Design review of the part built by this model. Coordinates are the model's own, in mm. Coordinates: 2 decimals unless noted, no trailing zeros. Use a Markdown table: item, result.
from build123d import *

# Parameters (mm, degrees)
F0_R     = 47.625
F0_R_2   = 1.5875
F0_R_3   = 19.05
F0_R_4   = 14.2875
F1_DEPTH = 3.175
F2_DEPTH = 12.7
F3_SIZE  = 3.17499
F4_SIZE  = 0.79375
F5_SIZE  = 0.79375
F6_R     = 5.08
F7_SIZE  = 3.175


# Not quite as in the source:
# - a fillet or chamfer is up to 0.001 mm smaller than in the source, because OpenCascade refuses the exact size


with BuildPart() as f1:
    # F0 (on Front) → F1 (new body)
    with BuildSketch(Plane.XZ):
        Circle(F0_R)
        with Locations((0, -34.925)):
            Circle(F0_R_2, mode=Mode.SUBTRACT)
        with Locations((-34.925, 0)):
            Circle(F0_R_2, mode=Mode.SUBTRACT)
        Circle(F0_R_3, mode=Mode.SUBTRACT)
        with Locations((34.925, 0)):
            Circle(F0_R_2, mode=Mode.SUBTRACT)
        with Locations((0, 34.925)):
            Circle(F0_R_2, mode=Mode.SUBTRACT)
        Circle(F0_R_3)
        Circle(F0_R_4, mode=Mode.SUBTRACT)
    extrude(amount=F1_DEPTH)

    # F0 (on Front) → F2 (join)
    with BuildSketch(Plane.XZ):
        Circle(F0_R_3)
        Circle(F0_R_4, mode=Mode.SUBTRACT)
    extrude(amount=F2_DEPTH)

    # F3 (size 3.175 in the source; OpenCascade refuses exactly that, so slightly less here)
    f3_edges = [f1.edges().sort_by_distance(p)[0] for p in [
        (-1.5875, -3.175, 34.925),
        (-36.5125, -3.175, 0),
        (33.3375, -3.175, 0),
        (-1.5875, -3.175, -34.925),
    ]]
    chamfer(f3_edges, length=F3_SIZE)

    # F4
    f4_edges = [f1.edges().sort_by_distance(p)[0] for p in [
        (-47.625, -3.175, 0),
    ]]
    chamfer(f4_edges, length=F4_SIZE)

    # F5
    f5_edges = [f1.edges().sort_by_distance(p)[0] for p in [
        (-19.05, -12.7, 0),
        (-14.2875, -12.7, 0),
    ]]
    chamfer(f5_edges, length=F5_SIZE)

    # F6
    f6_edges = [f1.edges().sort_by_distance(p)[0] for p in [
        (-19.05, -3.175, 0),
    ]]
    fillet(f6_edges, radius=F6_R)

    # F7
    f7_edges = [f1.edges().sort_by_distance(p)[0] for p in [
        (-14.2875, 0, 0),
    ]]
    chamfer(f7_edges, length=F7_SIZE)


solid = f1.part
(1) For pin 1 (2.5 mm diameter, centred on x = -34.925, z = 0, fed in from -Y); pin 2 (1.5 mm diameter, centred on x = 17.5, z = 28, fed in from -Y) (3 decimals); pin 3 (4 mm diameter, centred on x = 31, y = -3, fed in from +Z); pin 4 (2 mm diameter, centred on x = 8, y = -8, fed in from +Z), all flat-tipped, find the tip position at first contact; note any pin that passes through.
Determined:
| item | result |
|---|---|
| pin 1 | through |
| pin 2 | y = -3.175 |
| pin 3 | z = 37.7 |
| pin 4 | z = 17.73 |
(2) Take a section at A-A on z = 0. State how many separate pieces and enclosed holes the cut face has, and give its area (3 significant figures).
Determined:
| item | result |
|---|---|
| separate pieces | 4 |
| enclosed holes | 0 |
| area | 261 mm2 |
(3) Draft analysis for pull direction X (two halves, no side actions). For faces 1 (the cylindrical face through (-15.12, -10.06, -11.59)), 2 (the flat face through (20, -3.175, -20)), 3 (the conical face through (-3.14, -2.98, -14.14)), state which applies: +X half, -X half, draft (parallel to the pull), parting line (faces both ways), or undercut.
Determined:
| item | result |
|---|---|
| face 1 | parting line |
| face 2 | draft |
| face 3 | undercut |
(4) For L1, parallel to Y at x = -8.5, z = 37.5 (3 decimals); L2, parallel to Z at x = 0, y = -8.5; L3, parallel to X at y = -2.25, z = 33, list the stretches that pass through material, from the lowest coordinate up. Write a range as from..to.
Determined:
| item | result |
|---|---|
| L1 | -3.175..0 |
| L2 | -19.05..-14.29, 14.29..19.05 |
| L3 | -34.34..-3.32, 3.32..34.34 |
